Source: CAD feature listing. Evaluate the final solid. Frame: model axes, mm. Coordinates: 2 decimals unless noted, no trailing zeros. Write each loop counter-clockwise with the first axis right and the second up, starting at its lowest first coordinate (ties: lowest second). Pieces come first, ordered by that corner, then holes. Notation, with made-up numbers: M -39.5,-31 L -29.5,-31 A25 ccw -29.5,2 Z; hole C 2.25,17.5 d2. An arc over 180 degrees is marked long. Answer as CSV lines item,"result". Start each with the question number.
1. Line query: probe 1 along X at (y, z) = (-9, -0.5); probe 2 along X at (y, z) = (-10, 1); probe 3 along Y at (x, z) = (-109, -3). Output: solid intervals per line, ascending. Write a range as [from, to].
2. Section B-B on x = 57. Return the cut outline in (y, z) (3 decimals), plus the area to 3 significant figures.
3. Contact query for flat-ended pins moving along their axis: pin 1 Ø1.9 at (x, z) = (48, 0) entering from -Y (3 decimals); pin 2 Ø12 at (x, y) = (-97, -14) entering from -Z; pin 3 Ø1.9 at (y, z) = (-13, -1.5) entering from +X; pin 4 Ø3 at (y, z) = (10, -1) entering from +X. Output: stop coordinate, or through.
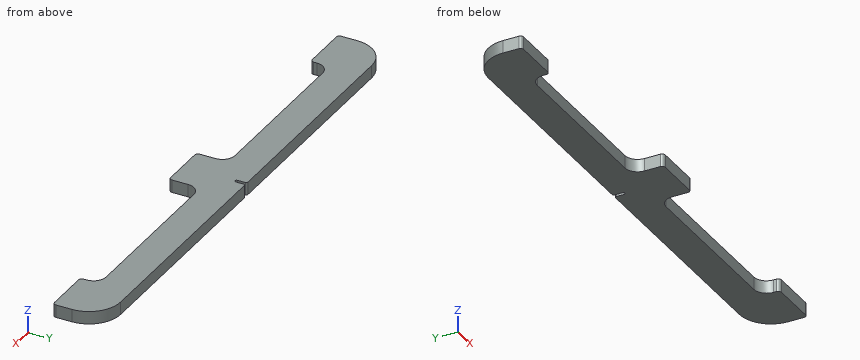
```python
from build123d import *

# Parameters (mm, degrees)
SKETCH1_W           = 25.4
SKETCH1_H           = 6.35
EXTRUDE1_DEPTH      = 131.7625
EXTRUDE2_REACH      = 134.525
FILLET1_R           = 15.875
SKETCH3_W           = 25.4
SKETCH3_H           = 6.35
TAB1_DEPTH          = 6.35
BREAK_CORNER1_START = -3.175
BREAK_CORNER1_DEPTH = 6.35
CUT_EXTRUDE1_REACH  = 135.284
FILLET2_R           = 0.79375


# Read off the part's stored shape, not the designer's step: Break-Corner1
# Sheet-metal steps are written as plain solids
with BuildPart() as part:
    # Sketch1 → Extrude1 (new, symmetric)
    with BuildSketch(Plane.YZ):
        Rectangle(SKETCH1_W, SKETCH1_H)
    extrude(amount=EXTRUDE1_DEPTH, both=True)

    # Sketch2 → Extrude2 (cut, up to next)
    with BuildSketch(Plane.XY.offset(3.175), mode=Mode.PRIVATE) as extrude2_sk1:
        with BuildLine():
            Line((-106.3625, -12.7), (-12.7, -12.7))
            Line((-12.7, -12.7), (-12.7, -9.525))
            ThreePointArc((-12.7, -9.525), (-14.559871939, -5.034871939), (-19.05, -3.175))
            Line((-19.05, -3.175), (-100.0125, -3.175))
            ThreePointArc((-100.0125, -3.175), (-104.502628061, -5.034871939), (-106.3625, -9.525))
            Line((-106.3625, -9.525), (-106.3625, -12.7))
        make_face()
    extrude2_tool1 = extrude(extrude2_sk1.sketch, amount=-EXTRUDE2_REACH, mode=Mode.PRIVATE) & part.part
    # Sketch2 → Extrude2 (cut, up to next)
    with BuildSketch(Plane.XY.offset(3.175), mode=Mode.PRIVATE) as extrude2_sk2:
        with BuildLine():
            Line((12.7, -12.7), (106.3625, -12.7))
            Line((106.3625, -12.7), (106.3625, -9.525))
            ThreePointArc((106.3625, -9.525), (104.502628061, -5.034871939), (100.0125, -3.175))
            Line((100.0125, -3.175), (19.05, -3.175))
            ThreePointArc((19.05, -3.175), (14.559871939, -5.034871939), (12.7, -9.525))
            Line((12.7, -9.525), (12.7, -12.7))
        make_face()
    extrude2_tool2 = extrude(extrude2_sk2.sketch, amount=-EXTRUDE2_REACH, mode=Mode.PRIVATE) & part.part
    add(extrude2_tool1.solids().sort_by_distance((-59.53125, -8.003656, 3.175))[0], mode=Mode.SUBTRACT)
    add(extrude2_tool2.solids().sort_by_distance((59.53125, -8.003656, 3.175))[0], mode=Mode.SUBTRACT)

    # Fillet1
    fillet1_edges = [part.edges().sort_by_distance(p)[0] for p in [
        (131.7625, 12.7, 0),
        (-131.7625, 12.7, 0),
    ]]
    fillet(fillet1_edges, radius=FILLET1_R)

    # Sketch3 → Tab1 (add)
    with BuildSketch(Plane(origin=(0, 0, -3.175), x_dir=(-1, 0, 0), z_dir=(0, 0, -1))):
        with Locations((0, -15.875)):
            Rectangle(SKETCH3_W, SKETCH3_H)
    extrude(amount=-TAB1_DEPTH)

    # Break-Corner1 outline → Break-Corner1 (cut)
    with BuildSketch(Plane.XY.offset(BREAK_CORNER1_START)):
        with BuildLine():
            Line((-131.7625, -12.7), (-130.175, -12.7))
            ThreePointArc((-130.175, -12.7), (-131.297532015, -12.235032015), (-131.7625, -11.1125))
            Line((-131.7625, -11.1125), (-131.7625, -12.7))
        make_face()
        with BuildLine():
            ThreePointArc((-106.3625, -11.1125), (-106.827467985, -12.235032015), (-107.95, -12.7))
            Line((-107.95, -12.7), (-106.3625, -12.7))
            Line((-106.3625, -12.7), (-106.3625, -11.1125))
        make_face()
        with BuildLine():
            ThreePointArc((12.7, -17.4625), (12.235032015, -18.585032015), (11.1125, -19.05))
            Line((11.1125, -19.05), (12.7, -19.05))
            Line((12.7, -19.05), (12.7, -17.4625))
        make_face()
        with BuildLine():
            ThreePointArc((-11.1125, -19.05), (-12.235032015, -18.585032015), (-12.7, -17.4625))
            Line((-12.7, -17.4625), (-12.7, -19.05))
            Line((-12.7, -19.05), (-11.1125, -19.05))
        make_face()
        with BuildLine():
            Line((106.3625, -12.7), (107.95, -12.7))
            ThreePointArc((107.95, -12.7), (106.827467985, -12.235032015), (106.3625, -11.1125))
            Line((106.3625, -11.1125), (106.3625, -12.7))
        make_face()
        with BuildLine():
            ThreePointArc((131.7625, -11.1125), (131.297532015, -12.235032015), (130.175, -12.7))
            Line((130.175, -12.7), (131.7625, -12.7))
            Line((131.7625, -12.7), (131.7625, -11.1125))
        make_face()
    extrude(amount=BREAK_CORNER1_DEPTH, mode=Mode.SUBTRACT)

    # Sketch4 → Cut-Extrude1 (cut, up to next)
    with BuildSketch(Plane(origin=(0, 0, -3.175), x_dir=(-1, 0, 0), z_dir=(0, 0, -1)), mode=Mode.PRIVATE) as cut_extrude1_sk1:
        with BuildLine():
            Line((0.79375, 12.7), (0.79375, 7.9375))
            ThreePointArc((0.79375, 7.9375), (0, 7.14375), (-0.79375, 7.9375))
            Line((-0.79375, 7.9375), (-0.79375, 12.7))
            ThreePointArc((-0.79375, 12.7), (0, 13.49375), (0.79375, 12.7))
        make_face()
    cut_extrude1_tool1 = extrude(cut_extrude1_sk1.sketch, amount=-CUT_EXTRUDE1_REACH, mode=Mode.PRIVATE) & part.part
    add(cut_extrude1_tool1.solids().sort_by_distance((0, 10.31875, -3.175))[0], mode=Mode.SUBTRACT)

    # Fillet2
    fillet2_edges = [part.edges().sort_by_distance(p)[0] for p in [
        (-0.79375, 12.7, 0),
        (0.79375, 12.7, 0),
    ]]
    fillet(fillet2_edges, radius=FILLET2_R)


solid = part.part
```
Values:
1,probe 1,"[-131.76, -106.34], [-12.72, 12.72], [106.34, 131.76]"
1,probe 2,"[-131.76, -106.36], [-12.7, 12.7], [106.36, 131.76]"
1,probe 3,"[-12.7, 12.7]"
2,outline,"M -3.175,-3.175 L 12.7,-3.175 L 12.7,3.175 L -3.175,3.175 Z"
2,area,"101 mm²"
3,pin 1,"y = -3.175"
3,pin 2,"through"
3,pin 3,"x = 131.46"
3,pin 4,"x = 126.64"
